from build123d import *

# Parameters (mm, degrees)
RESSALTO_EXTRUS_O1_DEPTH = 54.6
ESBO_O2_R                = 3.98
CORTE_EXTRUS_O1_DEPTH    = 212.979645249


with BuildPart() as part:
    # Esboço1 → Ressalto-extrusão1 (new body)
    with BuildSketch(Plane(origin=(0, 0, 0), x_dir=(0, 0, -1), z_dir=(1, 0, 0))):
        Polygon((0, 0), (25, 0), (25, 152.8), (10, 152.8), (10, 153.9), (10, 155), (26.1, 155), (133.9, 155), (150, 155), (150, 152.8), (135, 152.8), (135, 0), (158.9, 0), (158.9, -1.1), (133.9, -1.1), (133.9, 153.9), (26.1, 153.9), (26.1, -1.1), (0, -1.1), align=None)
    extrude(amount=RESSALTO_EXTRUS_O1_DEPTH)

    # Esboço2 → Corte-extrusão1 (cut, through all)
    with BuildSketch(Plane.XY.offset(-25)):
        with Locations((26.9, 6)):
            Circle(ESBO_O2_R)
        with Locations((48.4, 18.7)):
            Circle(ESBO_O2_R)
        with Locations((26.9, 31.4)):
            Circle(ESBO_O2_R)
        with Locations((48.4, 44.1)):
            Circle(ESBO_O2_R)
        with Locations((26.9, 56.8)):
            Circle(ESBO_O2_R)
        with Locations((48.4, 69.5)):
            Circle(ESBO_O2_R)
        with Locations((26.9, 82.2)):
            Circle(ESBO_O2_R)
        with Locations((48.4, 94.9)):
            Circle(ESBO_O2_R)
        with Locations((26.9, 107.6)):
            Circle(ESBO_O2_R)
        with Locations((48.4, 120.3)):
            Circle(ESBO_O2_R)
        with Locations((26.9, 133)):
            Circle(ESBO_O2_R)
        with Locations((48.4, 145.7)):
            Circle(ESBO_O2_R)
    extrude(amount=-CORTE_EXTRUS_O1_DEPTH, mode=Mode.SUBTRACT)


solid = part.part
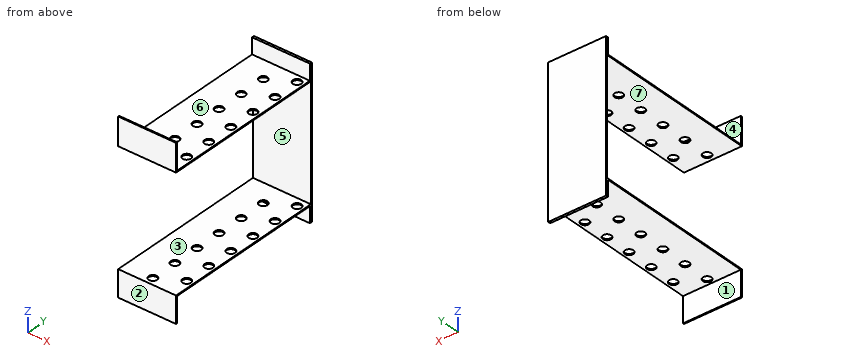
Build history of the part. All positions in model axes, mm. Face numbers are marked on the shaded views. A direction names the side the tool comes from. Round coordinates to 2 decimals unless told otherwise and drop trailing zeros. Loops run counter-clockwise (first coordinate to the right, second up) from the corner with the lowest first, then second, coordinate; pieces in that order, holes last. Notation, with made-up numbers: (17, 58) -> (37, 58) arc R8 ccw to (37, 63) -> close; hole circle Ø11 at (26.25, 29.5). An arc over 180 degrees is marked (long way). Answer in a Markdown table with one row per item.
Item 1: Which spindle directions (+Z, -Z, +X, -X, +Y, -Y) get a long thin tool onto all of the face, cutting with end or side? Do the marked faces 1, 2 and 3. Say none if no direction does.
Answers below:
| item | result |
|---|---|
| face 1 | -Z, +X, -X |
| face 2 | +Z, -Z, +X, -X, -Y |
| face 3 | +X, -X, -Y |
Item 2: Mould opens along Y. For the marked faces 4, 5, 6 and 7 say: +Y half, -Y half, draft (parallel to the pull), parting line (faces both ways), or undercut.
Answers below:
| item | result |
|---|---|
| face 4 | undercut |
| face 5 | -Y half |
| face 6 | undercut |
| face 7 | draft |
Item 3: Drill centre lines: L1, parallel to Z at x = 6, y = 85; L2, parallel to Y at x = 29, z = -147; L3, parallel to Y at x = 26, z = -77. Where is each one in solid material? Low to high. Write a range as [from, to].
Answers below:
| item | result |
|---|---|
| L1 | z = [-135, -133.9], [-26.1, -25] |
| L2 | y = [-1.1, 0], [152.8, 155] |
| L3 | y = [153.9, 155] |
Item 4: Pin check, flat tips, straight feed: pin 1 (1.1 mm diameter, centred on x = 25, y = 153.5, fed in from +Z); pin 2 (12 mm diameter, centred on x = 12, y = 97, fed in from +Z); pin 3 (5 mm diameter, centred on x = 48.4, y = 44.1, fed in from +Z); pin 4 (1.5 mm diameter, centred on x = 10.5, z = -103, fed in from -Y). Stop position of each tip, or through.
Answers below:
| item | result |
|---|---|
| pin 1 | stops at z = -10 |
| pin 2 | stops at z = -25 |
| pin 3 | passes through |
| pin 4 | stops at y = 153.9 |
Item 5: Saw through at D-D (x = 48.4). State how many separate pieces and enclosed holes the cut face has, and give its area (3 significant figures).
Answers below:
| item | result |
|---|---|
| separate pieces | 13 |
| enclosed holes | 0 |
| area | 477 mm² |
Item 6: Saw through at B-B (x = 39). Write the cut outline in (y, z), and give its area (3 significant figures).
Answers below:
| item | result |
|---|---|
| outline | (-1.1, -158.9) -> (0, -158.9) -> (0, -135) -> (152.8, -135) -> (152.8, -150) -> (155, -150) -> (155, -10) -> (152.8, -10) -> (152.8, -25) -> (0, -25) -> (0, 0) -> (-1.1, 0) -> (-1.1, -26.1) -> (153.9, -26.1) -> (153.9, -133.9) -> (-1.1, -133.9) -> close |
| area | 582 mm² |
Item 7: Saw through at C-C (z = -106.5). Write the cut outline in (x, y), and give its area (3 significant figures).
Answers below:
| item | result |
|---|---|
| outline | (0, 153.9) -> (54.6, 153.9) -> (54.6, 155) -> (0, 155) -> close |
| area | 60.1 mm² |
Item 8: Saw through at A-A (y = 133). Write the cut outline in (x, z), and give its area (3 significant figures).
Answers below:
| item | result |
|---|---|
| outline | (0, -135) -> (22.92, -135) -> (22.92, -133.9) -> (0, -133.9) -> close; (0, -26.1) -> (22.92, -26.1) -> (22.92, -25) -> (0, -25) -> close; (30.88, -135) -> (54.6, -135) -> (54.6, -133.9) -> (30.88, -133.9) -> close; (30.88, -26.1) -> (54.6, -26.1) -> (54.6, -25) -> (30.88, -25) -> close |
| area | 103 mm² |
